from build123d import *

# Parameters (mm, degrees)
CROQUIS1_W               = 38
CROQUIS1_H               = 81
CROQUIS1_W_2             = 27
CROQUIS1_H_2             = 72
CROQUIS1_H_3             = 38
CROQUIS1_R               = 3.5
SALIENTE_EXTRUIR1_DEPTH  = 5
CROQUIS2_W               = 38
CROQUIS2_H               = 81
CROQUIS2_W_2             = 27
CROQUIS2_H_2             = 72
SALIENTE_EXTRUIR2_DEPTH  = 5
SALIENTE_EXTRUIR9_START  = -1
SALIENTE_EXTRUIR9_DEPTH  = 1
SALIENTE_EXTRUIR10_DEPTH = 11
SALIENTE_EXTRUIR11_DEPTH = 10
REDONDEO1_R              = 1
REDONDEO2_R              = 1
REDONDEO3_R              = 1
CROQUIS6_W               = 6
CROQUIS6_H               = 9
CORTAR_EXTRUIR1_DEPTH    = 8
CROQUIS7_W               = 6
CROQUIS7_H               = 9
CROQUIS7_R               = 2.5
SALIENTE_EXTRUIR12_DEPTH = 3
SALIENTE_EXTRUIR13_DEPTH = 11
REDONDEO4_R              = 5
CROQUIS9_R               = 0.6
CORTAR_EXTRUIR2_DEPTH    = 80
SALIENTE_EXTRUIR14_START = -2.5
CROQUIS10_R              = 0.6
SALIENTE_EXTRUIR14_DEPTH = 2.5
CROQUIS11_R              = 4
CROQUIS11_R_2            = 3.5
CROQUIS11_R_3            = 2.5
CROQUIS11_R_4            = 2
CORTAR_EXTRUIR3_DEPTH    = 1
SALIENTE_EXTRUIR15_DEPTH = 3
CROQUIS14_R              = 1.5
CORTAR_EXTRUIR4_DEPTH    = 14
CROQUIS16_W              = 3.5
CROQUIS16_H              = 3
SALIENTE_EXTRUIR16_DEPTH = 4
CROQUIS25_R              = 3
CROQUIS25_R_2            = 1.5
SALIENTE_EXTRUIR21_DEPTH = 18
CROQUIS26_R              = 1.5
CORTAR_EXTRUIR7_DEPTH    = 18
CROQUIS28_R              = 1
CORTAR_EXTRUIR8_DEPTH    = 4
CROQUIS29_R              = 3
CROQUIS29_R_2            = 1.5
CORTAR_EXTRUIR9_DEPTH    = 5
CROQUIS31_W              = 16
CROQUIS31_H              = 4
CORTAR_EXTRUIR10_DEPTH   = 5


with BuildPart() as part:
    # Croquis1 → Saliente-Extruir1 (new body)
    # profile 1 of 5: a face of its own
    with BuildSketch(Plane.XY):
        Rectangle(CROQUIS1_W, CROQUIS1_H)
        Rectangle(CROQUIS1_W_2, CROQUIS1_H_2, mode=Mode.SUBTRACT)
    # profile 2 of 5: a face of its own
    with BuildSketch(Plane.XY):
        with Locations((0, -59.5)):
            Rectangle(CROQUIS1_W, CROQUIS1_H_3)
        with Locations((-9.5, -69)):
            Circle(CROQUIS1_R, mode=Mode.SUBTRACT)
        with Locations((9.5, -59.5)):
            Circle(CROQUIS1_R, mode=Mode.SUBTRACT)
        with Locations((-9.5, -50)):
            Circle(CROQUIS1_R, mode=Mode.SUBTRACT)
    # profile 3 of 5: a face of its own
    with BuildSketch(Plane.XY):
        with BuildLine():
            ThreePointArc((19, -78.5), (26.870057685, -59.5), (19, -40.5))
            Line((19, -40.5), (19, -78.5))
        make_face()
    # profile 4 of 5: a face of its own
    with BuildSketch(Plane.XY):
        with BuildLine():
            Line((19, -78.5), (-19, -78.5))
            ThreePointArc((-19, -78.5), (0, -86.370057685), (19, -78.5))
        make_face()
    # profile 5 of 5: a face of its own
    with BuildSketch(Plane.XY):
        with BuildLine():
            Line((-19, -78.5), (-19, -40.5))
            ThreePointArc((-19, -40.5), (-26.870057685, -59.5), (-19, -78.5))
        make_face()
    extrude(amount=SALIENTE_EXTRUIR1_DEPTH)

    # Croquis2 → Saliente-Extruir2 (add)
    with BuildSketch(Plane(origin=(0, 0, 0), x_dir=(-1, 0, 0), z_dir=(0, 0, -1))):
        Rectangle(CROQUIS2_W, CROQUIS2_H)
        Rectangle(CROQUIS2_W_2, CROQUIS2_H_2, mode=Mode.SUBTRACT)
    extrude(amount=SALIENTE_EXTRUIR2_DEPTH)

    # Croquis3 → Saliente-Extruir9 (add)
    with BuildSketch(Plane.XY.offset(5).offset(SALIENTE_EXTRUIR9_START)):
        with BuildLine():
            Line((26.870057685, -59.5), (26.870057685, 40.5))
            Line((26.870057685, 40.5), (19, 48.370057685))
            Line((19, 48.370057685), (-19, 48.370057685))
            Line((-19, 48.370057685), (-26.870057685, 40.5))
            Line((-26.870057685, 40.5), (-26.870057685, -59.5))
            ThreePointArc((-26.870057685, -59.5), (0, -86.370057685), (26.870057685, -59.5))
        make_face()
        with BuildLine():
            Line((19, -59.5), (19, 40.5))
            Line((19, 40.5), (-19, 40.5))
            Line((-19, 40.5), (-19, -59.5))
            ThreePointArc((-19, -59.5), (0, -78.5), (19, -59.5))
        make_face(mode=Mode.SUBTRACT)
    extrude(amount=SALIENTE_EXTRUIR9_DEPTH)

    # Croquis4 → Saliente-Extruir10 (add)
    with BuildSketch(Plane(origin=(0, 0, 4), x_dir=(-1, 0, 0), z_dir=(0, 0, -1))):
        with BuildLine():
            Line((19, 40.5), (19, -40.5))
            ThreePointArc((19, -40.5), (24.824696333, -49.217274097), (26.870057685, -59.5))
            Line((26.870057685, -59.5), (26.870057685, 40.5))
            Line((26.870057685, 40.5), (19, 48.370057685))
            Line((19, 48.370057685), (-19, 48.370057685))
            Line((-19, 48.370057685), (-26.870057685, 40.5))
            Line((-26.870057685, 40.5), (-26.870057685, -59.5))
            ThreePointArc((-26.870057685, -59.5), (-24.824696333, -49.217274097), (-19, -40.5))
            Line((-19, -40.5), (-19, 40.5))
            Line((-19, 40.5), (19, 40.5))
        make_face()
    extrude(amount=-SALIENTE_EXTRUIR10_DEPTH)

    # Croquis5 → Saliente-Extruir11 (add)
    with BuildSketch(Plane.XY.offset(5)):
        with BuildLine():
            Line((-19, -59.5), (-19, -69))
            ThreePointArc((-19, -69), (-16.217514421, -75.717514421), (-9.5, -78.5))
            Line((-9.5, -78.5), (9.5, -78.5))
            ThreePointArc((9.5, -78.5), (16.217514421, -75.717514421), (19, -69))
            Line((19, -69), (19, -59.5))
            Line((19, -59.5), (19, -40.5))
            ThreePointArc((19, -40.5), (0, -86.370057685), (-19, -40.5))
            Line((-19, -40.5), (-19, -59.5))
        make_face()
    extrude(amount=SALIENTE_EXTRUIR11_DEPTH)

    # Redondeo1
    redondeo1_edges = [part.edges().sort_by_distance(p)[0] for p in [
        (19, -40.5, -2.5),
        (-19, -40.5, -2.5),
        (19, 40.5, -0.5),
        (-19, 40.5, -0.5),
    ]]
    fillet(redondeo1_edges, radius=REDONDEO1_R)

    # Redondeo2
    redondeo2_edges = [part.edges().sort_by_distance(p)[0] for p in [
        (-19, -0.5, 4),
        (0, 40.5, 4),
        (-18.707106781, 40.207106781, 4),
        (18.707106781, 40.207106781, 4),
        (19, -0.5, 4),
    ]]
    fillet(redondeo2_edges, radius=REDONDEO2_R)

    # Redondeo3
    redondeo3_edges = [part.edges().sort_by_distance(p)[0] for p in [
        (19, 48.370057685, 9.5),
        (26.870057685, 40.5, 9.5),
        (-26.870057685, 40.5, 9.5),
        (-19, 48.370057685, 9.5),
    ]]
    fillet(redondeo3_edges, radius=REDONDEO3_R)

    # Croquis6 → Cortar-Extruir1 (cut)
    with BuildSketch(Plane.ZY.offset(26.870057685)):
        with Locations((11.5, -55)):
            Rectangle(CROQUIS6_W, CROQUIS6_H)
    extrude(amount=-CORTAR_EXTRUIR1_DEPTH, mode=Mode.SUBTRACT)

    # Croquis7 → Saliente-Extruir12 (add)
    with BuildSketch(Plane.ZY.offset(26.870057685)):
        with Locations((11.5, -55)):
            Rectangle(CROQUIS7_W, CROQUIS7_H)
        with Locations((11.5, -55)):
            Circle(CROQUIS7_R, mode=Mode.SUBTRACT)
    extrude(amount=-SALIENTE_EXTRUIR12_DEPTH)

    # Croquis8 → Saliente-Extruir13 (add)
    with BuildSketch(Plane.ZY.offset(26.870057685)):
        Polygon((15, 40.085786438), (4, 40.085786438), (4, 37.085786438), (9.5, 37.085786438), (15, 37.085786438), align=None)
        Polygon((9.5, 15.085786438), (4, 15.085786438), (4, 12.085786438), (9.5, 12.085786438), (15, 12.085786438), (15, 15.085786438), align=None)
        Polygon((9.5, -10.914213562), (4, -10.914213562), (4, -13.914213562), (9.5, -13.914213562), (15, -13.914213562), (15, -10.914213562), align=None)
        Polygon((9.5, -36.914213562), (4, -36.914213562), (4, -39.914213562), (15, -39.914213562), (15, -36.914213562), align=None)
    extrude(amount=SALIENTE_EXTRUIR13_DEPTH)

    # Redondeo4
    redondeo4_edges = [part.edges().sort_by_distance(p)[0] for p in [
        (-37.870057685, 38.585786438, 4),
        (-37.870057685, 38.585786438, 15),
        (-37.870057685, 13.585786438, 4),
        (-37.870057685, 13.585786438, 15),
        (-37.870057685, -12.414213562, 4),
        (-37.870057685, -12.414213562, 15),
        (-37.870057685, -38.414213562, 4),
        (-37.870057685, -38.414213562, 15),
    ]]
    fillet(redondeo4_edges, radius=REDONDEO4_R)

    # Croquis9 → Cortar-Extruir2 (cut)
    with BuildSketch(Plane(origin=(0, 40.085786438, 0), x_dir=(1, 0, 0), z_dir=(0, 1, 0))):
        with Locations(Location((-32.370057685, -9.5, 0), (0, 0, 270))):
            Circle(CROQUIS9_R)
    extrude(amount=-CORTAR_EXTRUIR2_DEPTH, mode=Mode.SUBTRACT)

    # Croquis10 → Saliente-Extruir14 (add)
    with BuildSketch(Plane.XZ.offset(39.914213562).offset(SALIENTE_EXTRUIR14_START)):
        with Locations(Location((-32.370057685, 9.5, 0), (0, 0, 90))):
            Circle(CROQUIS10_R)
    extrude(amount=SALIENTE_EXTRUIR14_DEPTH)

    # Croquis11 → Cortar-Extruir3 (cut)
    # profile 1 of 2: a face of its own
    with BuildSketch(Plane(origin=(0, -36.914213562, 0), x_dir=(1, 0, 0), z_dir=(0, 1, 0))):
        with Locations(Location((-32.370057685, -9.5, 0), (0, 0, 270))):
            Circle(CROQUIS11_R)
        with Locations(Location((-32.370057685, -9.5, 0), (0, 0, 270))):
            Circle(CROQUIS11_R_2, mode=Mode.SUBTRACT)
    # profile 2 of 2: a face of its own
    with BuildSketch(Plane(origin=(0, -36.914213562, 0), x_dir=(1, 0, 0), z_dir=(0, 1, 0))):
        with Locations(Location((-32.370057685, -9.5, 0), (0, 0, 270))):
            Circle(CROQUIS11_R_3)
        with Locations(Location((-32.370057685, -9.5, 0), (0, 0, 270))):
            Circle(CROQUIS11_R_4, mode=Mode.SUBTRACT)
    extrude(amount=-CORTAR_EXTRUIR3_DEPTH, mode=Mode.SUBTRACT)

    # Croquis13 → Saliente-Extruir15 (add)
    with BuildSketch(Plane.XY.offset(15)):
        Polygon((-19, -65.5), (-19, 40.5), (-22.5, 40.5), (-22.5, -69), (-19, -69), align=None)
        Polygon((22.5, 40.5), (19, 40.5), (19, -65.5), (19, -69), (22.5, -69), align=None)
        with BuildLine():
            Line((-19, 40.5), (19, 40.5))
            Line((19, 40.5), (22.5, 40.5))
            Line((22.5, 40.5), (22.5, 44.870057685))
            Line((22.5, 44.870057685), (19.292893219, 48.077164466))
            ThreePointArc((19.292893219, 48.077164466), (18.96846987, 48.293937218), (18.585786438, 48.370057685))
            Line((18.585786438, 48.370057685), (-18.585786438, 48.370057685))
            ThreePointArc((-18.585786438, 48.370057685), (-18.96846987, 48.293937218), (-19.292893219, 48.077164466))
            Line((-19.292893219, 48.077164466), (-22.5, 44.870057685))
            Line((-22.5, 44.870057685), (-22.5, 40.5))
            Line((-22.5, 40.5), (-19, 40.5))
        make_face()
    extrude(amount=SALIENTE_EXTRUIR15_DEPTH)

    # Croquis14 → Cortar-Extruir4 (cut)
    with BuildSketch(Plane(origin=(0, 0, 4), x_dir=(-1, 0, 0), z_dir=(0, 0, -1))):
        with Locations((10, 45.370057685)):
            Circle(CROQUIS14_R)
        with Locations(Location((-10, 45.370057685, 0), (0, 0, 180))):
            Circle(CROQUIS14_R)
    extrude(amount=-CORTAR_EXTRUIR4_DEPTH, mode=Mode.SUBTRACT)

    # Croquis16 → Saliente-Extruir16 (add)
    with BuildSketch(Plane(origin=(0, -69, 0), x_dir=(-1, 0, 0), z_dir=(0, -1, 0))):
        with Locations((20.75, -16.5)):
            Rectangle(CROQUIS16_W, CROQUIS16_H)
        with Locations((-20.75, -16.5)):
            Rectangle(CROQUIS16_W, CROQUIS16_H)
    extrude(amount=SALIENTE_EXTRUIR16_DEPTH)

    # Croquis25 → Saliente-Extruir21 (add)
    with BuildSketch(Plane.XY.offset(18)):
        with Locations((0, -70.629942315)):
            Circle(CROQUIS25_R)
        with Locations((0, -70.629942315)):
            Circle(CROQUIS25_R_2, mode=Mode.SUBTRACT)
    extrude(amount=-SALIENTE_EXTRUIR21_DEPTH)

    # Croquis26 → Cortar-Extruir7 (cut)
    with BuildSketch(Plane.XY.offset(18)):
        with Locations((0, -70.629942315)):
            Circle(CROQUIS26_R)
    extrude(amount=-CORTAR_EXTRUIR7_DEPTH, mode=Mode.SUBTRACT)

    # Croquis28 → Cortar-Extruir8 (cut)
    with BuildSketch(Plane.XY.offset(5)):
        with Locations((-16.5, 38)):
            Circle(CROQUIS28_R)
        with Locations((14.5, 38)):
            Circle(CROQUIS28_R)
        with Locations((14.5, -37)):
            Circle(CROQUIS28_R)
        with Locations((-16.5, -37)):
            Circle(CROQUIS28_R)
    extrude(amount=-CORTAR_EXTRUIR8_DEPTH, mode=Mode.SUBTRACT)

    # Croquis29 → Cortar-Extruir9 (cut)
    with BuildSketch(Plane.XY.offset(18)):
        with Locations((0, -70.629942315)):
            Circle(CROQUIS29_R)
        with Locations((0, -70.629942315)):
            Circle(CROQUIS29_R_2, mode=Mode.SUBTRACT)
    extrude(amount=-CORTAR_EXTRUIR9_DEPTH, mode=Mode.SUBTRACT)

    # Croquis30 → Cortar-Revolución1 (revolve, cut)
    with BuildSketch(Plane.XY.offset(18)):
        Polygon((-1.8, 45.370057685), (-1.8, 40.5), (0.2, 40.5), (0.2, 48.370057685), (-1.8, 48.370057685), align=None)
    revolve(axis=Axis((-1.8, 45.370057685, 18), (0, -1, 0)), mode=Mode.SUBTRACT)

    # Croquis31 → Cortar-Extruir10 (cut)
    with BuildSketch(Plane.XY.offset(5)):
        with Locations((2, -42.5)):
            Rectangle(CROQUIS31_W, CROQUIS31_H)
    extrude(amount=-CORTAR_EXTRUIR10_DEPTH, mode=Mode.SUBTRACT)


solid = part.part
Read the model definition and answer for the solid it produces. Units are mm, in the model's axes. A direction names the side the tool comes from. Round coordinates to 2 decimals unless told otherwise and drop trailing zeros. Loops run counter-clockwise (first coordinate to the right, second up) from the corner with the lowest first, then second, coordinate; pieces in that order, holes last. Notation, with made-up numbers: (20.5, -16.5) - (45.5, -16.5) arc R28 ccw to (45.5, 16.5) - close; hole circle Ø1 at (48, -29.5). An arc over 180 degrees is marked (long way). One line per question, with ' | ' between items. Start each with the question number.
Q1. Find the intervals of material crossed by L1, parallel to Y at x = 0, z = 8; L2, parallel to Y at x = -9.5, z = 12; L3, parallel to Y at x = -10, z = 7.5, in increasing order.
Q2. For a pull along X with two mould halves and no side action, classify faces 6 (the flat face through (-31, 37.086, 9)), 7 (the flat face through (13.5, -1, 0)), 8 (the flat face through (-26.87, 1, 9)) as +X half, -X half, draft (parallel to the pull), parting line (faces both ways), or undercut.
Q3. Flat-ended cylindrical pins translate along their axes: pin 1 (3.5 mm diameter, centred on y = -16.5, z = 16.5, fed in from -X); pin 2 (5 mm diameter, centred on x = -1, z = -1.5, fed in from +Y); pin 3 (4 mm diameter, centred on x = -2.5, z = 10, fed in from -Y). Find the tip coordinate at first contact, or state that the pin passes through.
Q4. For faces 1 (the flat face through (0, -45, 5)), 2 (the flat face through (-22.5, -13, 17)), 3 (the flat face through (-36, -37.914, 9)), 4 (the flat face through (-26.87, -50, 9)), 5 (the flat face through (0, -40.5, -1)), determine the directions among +Z, -Z, +X, -X, +Y, -Y from which every point of the face is accessible in a straight line to the end or side of a thin tool.
Q5. Section A-A on y = -33 is taken. Give the vertices of the cut face in (x, z).
Established:
1) L1: -86.37 to -78.5, -73.63 to -72.13, -69.13 to -67.63, 40.5 to 48.37 | L2: -84.63 to -78.5, 40.5 to 43.96, 46.78 to 48.37 | L3: -84.44 to -78.49, 40.5 to 43.87, 46.87 to 48.37
2) face 6: draft | face 7: undercut | face 8: -X half
3) pin 1: x = -26.87 | pin 2: y = 40.5 | pin 3: y = -86.37
4) face 1: +Z | face 2: +Z, -X, +Y, -Y | face 3: none | face 4: +Z, -Z, -X, -Y | face 5: -Z
5) outline: (-26.87, 4) - (-20, 4) arc R1 cw to (-19, 3) - (-19, -5) - (-13.5, -5) - (-13.5, 5) - (-19, 5) - (-19, 18) - (-22.5, 18) - (-22.5, 15) - (-26.87, 15) - close; (13.5, -5) - (19, -5) - (19, 3) arc R1 cw to (20, 4) - (26.87, 4) - (26.87, 15) - (22.5, 15) - (22.5, 18) - (19, 18) - (19, 5) - (13.5, 5) - close
